Work out the finished part from the listing and answer in its coordinate system (mm). A direction names the side the tool comes from. Give positions to 0.01 mm unless a question says otherwise; leave off trailing zeros. Write each loop counter-clockwise with the first axis right and the second up, starting at its lowest first coordinate (ties: lowest second). Pieces come first, ordered by that corner, then holes. Notation, with made-up numbers: (6, -3) -> (38, -3) arc R34 cw to (38, 34) -> close; hole circle Ø10 at (7.5, 14). An arc over 180 degrees is marked (long way). Use a Markdown table: item, result. Add a question column.
Q1. For a pull along X with two mould halves and no side action, classify faces 1 (the face through (13.57, 1.02, 29.75)), 2 (the face through (-0.29, -7.27, 28.72)), 3 (the face through (-12, -5.608, 29)) as pulls with the +X half, pulls with the -X half, needs draft (parallel to the pull), parting line crosses it, or undercut.
Q2. Consider line 1 (Y direction, x = 0, z = 29.85); line 2 (X direction, y = 1.5, z = -16.25); line 3 (Y direction, x = 8.25, z = 0.5). Determine where each line is inside the solid, lowest interval first.
Q3. For faces 4 (the face through (-13.57, 1.02, 29.75)), 5 (the face through (7.845, -1, 22)), 6 (the face through (-10, -3, 29)), 7 (the face through (12, -0.5, 28)), 8 (the face through (-15, 1, -10)), determine the directions among +Z, -Z, +X, -X, +Y, -Y from which every point of the face is accessible in a straight line to the end or side of a thin tool.
Q4. Section C-C, the plane y = -24.5 is taken. Give the vertices of the cut face in (x, z), plus the area to 4 significant figures.
Q5. Section D-D, the plane x = 6 is taken. Give the vertices of the cut face in (y, z).
Q6. Section A-A, the plane z = -16.25 is taken. Give the vertices of the cut face in (x, y).
Q7. Section B-B, the plane x = 0 is taken. Give the vertices of the cut face in (y, z).
Q8. Each of these flat-tipped pins is pushed along its axis until it touches: pin 1 Ø8 at (x, y) = (-2.5, -33) entering from -Z; pin 2 Ø1.5 at (y, z) = (-2.5, 29) entering from -X; pin 3 Ø3 at (x, z) = (-7, -11.5) entering from -Y. Where does it stop, or does it pass through?
from build123d import *

# Parameters (mm, degrees)
SKETCH1_R               = 2.25
BOSS_EXTRUDE1_DEPTH     = 2.5
SKETCH3_R               = 2.25
SKETCH3_W               = 20
SKETCH3_H               = 2.5
BOSS_EXTRUDE2_DEPTH     = 5
BOSS_EXTRUDE3_DEPTH     = 3
SKETCH5_W               = 15.690952434
SKETCH5_H               = 6.78006253
BOSS_EXTRUDE4_DEPTH     = 10
CUT_EXTRUDE1_DEPTH      = 54.54884017
CUT_EXTRUDE1_DEPTH_BACK = 54.54884017
FILLET3_R               = 1


with BuildPart() as part:
    # Sketch1 → Boss-Extrude1 (new body)
    with BuildSketch(Plane(origin=(0, 0, 0), x_dir=(1, 0, 0), z_dir=(0, 1, 0))):
        with BuildLine():
            Line((15, 21.25), (15, -0.725838237))
            ThreePointArc((15, -0.725838237), (7.884185652, -13.487919119), (15, -26.25))
            Line((15, -26.25), (-15, -26.25))
            ThreePointArc((-15, -26.25), (-7.845476217, -13.487919119), (-15, -0.725838237))
            Line((-15, -0.725838237), (-15, 21.25))
            ThreePointArc((-15, 21.25), (-13.535533906, 24.785533906), (-10, 26.25))
            Line((-10, 26.25), (10, 26.25))
            ThreePointArc((10, 26.25), (13.535533906, 24.785533906), (15, 21.25))
        make_face()
        with Locations(Location((-7.5, 16.25, 0), (0, 0, 270))):
            Circle(SKETCH1_R, mode=Mode.SUBTRACT)
        with Locations(Location((7.5, 16.25, 0), (0, 0, 270))):
            Circle(SKETCH1_R, mode=Mode.SUBTRACT)
    extrude(amount=BOSS_EXTRUDE1_DEPTH)

    # Sketch3 → Boss-Extrude2 (add)
    # profile 1 of 2: a face of its own
    with BuildSketch(Plane.XY.offset(26.25)):
        with BuildLine():
            Line((10, 0), (-10, 0))
            Line((-10, 0), (-10, -5.607597834))
            Line((-10, -5.607597834), (-15, -5.607597834))
            Line((-15, -5.607597834), (-15, -32))
            ThreePointArc((-15, -32), (-13.535533906, -35.535533906), (-10, -37))
            Line((-10, -37), (10, -37))
            ThreePointArc((10, -37), (13.535533906, -35.535533906), (15, -32))
            Line((15, -32), (15, -5.607597834))
            Line((15, -5.607597834), (10, -5.607597834))
            Line((10, -5.607597834), (10, 0))
        make_face()
        with Locations((0, -24.5)):
            Circle(SKETCH3_R, mode=Mode.SUBTRACT)
        with Locations((0, -9.5)):
            Circle(SKETCH3_R, mode=Mode.SUBTRACT)
    # profile 2 of 2: a face of its own
    with BuildSketch(Plane.XY.offset(26.25)):
        with Locations((0, 1.25)):
            Rectangle(SKETCH3_W, SKETCH3_H)
    extrude(amount=BOSS_EXTRUDE2_DEPTH)

    # Sketch4 → Boss-Extrude3 (add)
    with BuildSketch(Plane(origin=(0, 2.5, 0), x_dir=(1, 0, 0), z_dir=(0, 1, 0))):
        with BuildLine():
            Line((10, -31.25), (10, -26.25))
            Line((10, -26.25), (15, -26.25))
            ThreePointArc((15, -26.25), (13.535533906, -29.785533906), (10, -31.25))
        make_face()
        with BuildLine():
            Line((-10, -31.25), (-10, -26.25))
            Line((-10, -26.25), (-15, -26.25))
            ThreePointArc((-15, -26.25), (-13.535533906, -29.785533906), (-10, -31.25))
        make_face()
    extrude(amount=-BOSS_EXTRUDE3_DEPTH)

    # Sketch5 → Boss-Extrude4 (add)
    with BuildSketch(Plane(origin=(0, 0, 26.25), x_dir=(-1, 0, 0), z_dir=(0, 0, -1))):
        with Locations((0, -3.390031265)):
            Rectangle(SKETCH5_W, SKETCH5_H)
    extrude(amount=BOSS_EXTRUDE4_DEPTH)

    # Sketch6 → Cut-Extrude1 (cut, two sides: drawn at the far end of the back side and taken through both)
    with BuildSketch(Plane(origin=(7.845476217, 0, 0), x_dir=(0, 0, -1), z_dir=(1, 0, 0)).offset(-CUT_EXTRUDE1_DEPTH_BACK)):
        with BuildLine():
            Line((-26.25, -6.78006253), (-24.66461888, -3.717189072))
            ThreePointArc((-24.66461888, -3.717189072), (-20.306619121, -2.19971294), (-16.25, 0))
            Line((-16.25, 0), (-16.25, -6.78006253))
            Line((-16.25, -6.78006253), (-26.25, -6.78006253))
        make_face()
    extrude(amount=CUT_EXTRUDE1_DEPTH + CUT_EXTRUDE1_DEPTH_BACK, mode=Mode.SUBTRACT)

    # Fillet3
    fillet3_edges = [part.edges().sort_by_distance(p)[0] for p in [
        (-7.845476217, -3.390031265, 26.25),
        (7.845476217, -3.390031265, 26.25),
    ]]
    fillet(fillet3_edges, radius=FILLET3_R)


solid = part.part
Result set:
| question | item | result |
|---|---|---|
| 1 | face 1 | pulls with the +X half |
| 1 | face 2 | undercut |
| 1 | face 3 | needs draft |
| 2 | line 1 | y = -37 to -26.75, -22.25 to -11.75, -7.25 to 2.5 |
| 2 | line 2 | x = -15 to -9.75, -5.25 to 5.25, 9.75 to 15 |
| 2 | line 3 | y = 0 to 2.5 |
| 3 | face 4 | +Z, -X, +Y |
| 3 | face 5 | -Z, +X, -Y |
| 3 | face 6 | +Z, -Z, -X |
| 3 | face 7 | +Z, -Z, +X |
| 3 | face 8 | +Z, -Z, -X, +Y, -Y |
| 4 | outline | (-15, 26.25) -> (-2.25, 26.25) -> (-2.25, 31.25) -> (-15, 31.25) -> close; (2.25, 26.25) -> (15, 26.25) -> (15, 31.25) -> (2.25, 31.25) -> close |
| 4 | area | 127.5 mm2 |
| 5 | outline | (-37, 26.25) -> (-6.78, 26.25) -> (-3.72, 24.66) arc R28.55 ccw to (0, 16.25) -> (0, -14.57) -> (2.5, -14.57) -> (2.5, 31.25) -> (-37, 31.25) -> close; (0, -26.25) -> (2.5, -26.25) -> (2.5, -17.93) -> (0, -17.93) -> close |
| 6 | outline | (-15, 0) -> (-9.75, 0) -> (-9.75, 2.5) -> (-15, 2.5) -> close; (-5.25, 0) -> (5.25, 0) -> (5.25, 2.5) -> (-5.25, 2.5) -> close; (9.75, 0) -> (15, 0) -> (15, 2.5) -> (9.75, 2.5) -> close |
| 7 | outline | (-37, 26.25) -> (-26.75, 26.25) -> (-26.75, 31.25) -> (-37, 31.25) -> close; (-22.25, 26.25) -> (-11.75, 26.25) -> (-11.75, 31.25) -> (-22.25, 31.25) -> close; (-7.25, 26.25) -> (-6.78, 26.25) -> (-3.72, 24.66) arc R28.55 ccw to (0, 16.25) -> (0, -26.25) -> (2.5, -26.25) -> (2.5, 31.25) -> (-7.25, 31.25) -> close |
| 8 | pin 1 | stops at z = 26.25 |
| 8 | pin 2 | stops at x = -10 |
| 8 | pin 3 | stops at y = 0 |
